```python
from build123d import *

# Parameters (mm, degrees)
F0_W     = 20
F0_H     = 20
F1_DEPTH = 20
F2_W     = 16
F2_H     = 16
F3_DEPTH = 16
F4_W     = 18
F4_H     = 18
F4_W_2   = 16
F4_H_2   = 16
F5_DEPTH = 4


with BuildPart() as f1:
    # F0 (on Right) → F1 (new body)
    with BuildSketch(Plane.YZ):
        Rectangle(F0_W, F0_H)
    extrude(amount=F1_DEPTH)

    # F2 (on face) → F3 (cut)
    with BuildSketch(Plane(origin=(0, 0, 0), x_dir=(0, -1, 0), z_dir=(-1, 0, 0))):
        Rectangle(F2_W, F2_H)
    extrude(amount=-F3_DEPTH, mode=Mode.SUBTRACT)

    # F4 (on face) → F5 (join)
    with BuildSketch(Plane(origin=(0, 0, 0), x_dir=(0, -1, 0), z_dir=(-1, 0, 0))):
        Rectangle(F4_W, F4_H)
        Rectangle(F4_W_2, F4_H_2, mode=Mode.SUBTRACT)
    extrude(amount=F5_DEPTH)


solid = f1.part
```
Can you work these out from the model? Positions are in its coordinate system, mm. A direction names the side the tool comes from. Round coordinates to 2 decimals unless told otherwise and drop trailing zeros. Loops run counter-clockwise (first coordinate to the right, second up) from the corner with the lowest first, then second, coordinate; pieces in that order, holes last.
Item 1: Suppose I cut it at A-A, the plane x = 13.5. Write out the boundary of the cut face in (y, z), then the cut area to 3 significant figures.
Item 2: Suppose I cut it at B-B, the plane z = 5.25. Write out the boundary of the cut face in (x, y), then the cut area to 3 significant figures.
Item 3: Which directions (+Z, -Z, +X, -X, +Y, -Y) give clear straight access to the entire face, cutting with the end or side of a thin tool? Please do faces 1 (the flat face through (-2, 0, 9)), 2 (the flat face through (6, 0, 8)), 3 (the flat face through (-2, 0, -9)), 4 (the flat face through (10, 10, 0)).
Item 4: Will these pins go through, and if not, where does the flat tip stop? pin 1 Ø12 at (y, z) = (-0.5, 6) entering from -X; pin 2 Ø8 at (y, z) = (0.5, -2) entering from -X; pin 3 Ø1.2 at (x, y) = (-1.5, -0.5) entering from -Z; pin 4 Ø2 at (x, y) = (-2.5, 0.5) entering from +Z.
Item 5: If we mould it in two halves opening along Y, with no side actions, what happens to faces 5 (the flat face through (-2, -9, 0)), 6 (the flat face through (6, -8, 0)), 7 (the flat face through (-2, 9, 0))? For each: +Y half, -Y half, draft (parallel to the pull), parting line (faces both ways), or undercut.
Item 6: Please list where these lines run through material, in increasing order: L1, parallel to Y at x = 10, z = -0.75; L2, parallel to Y at x = -1, z = 3.5.
Reported:
1. outline: (-10, -10) - (10, -10) - (10, 10) - (-10, 10) - close; hole (-8, -8) - (8, -8) - (8, 8) - (-8, 8) - close
1. area: 144 mm2
2. outline: (-4, -9) - (0, -9) - (0, -10) - (20, -10) - (20, 10) - (0, 10) - (0, 9) - (-4, 9) - (-4, 8) - (16, 8) - (16, -8) - (-4, -8) - close
2. area: 152 mm2
3. face 1: +Z, -X, +Y, -Y
3. face 2: -X
3. face 3: -Z, -X, +Y, -Y
3. face 4: +Z, -Z, +X, -X, +Y
4. pin 1: stops at x = -4
4. pin 2: stops at x = 16
4. pin 3: stops at z = -9
4. pin 4: stops at z = 9
5. face 5: -Y half
5. face 6: undercut
5. face 7: +Y half
6. L1: y = -10 to -8, 8 to 10
6. L2: y = -9 to -8, 8 to 9
